Part model, mm, in its own coordinate system. Face numbers are marked on the shaded views. A direction names the side the tool comes from. Give positions to 0.01 mm unless a question says otherwise; leave off trailing zeros. Write each loop counter-clockwise with the first axis right and the second up, starting at its lowest first coordinate (ties: lowest second). Pieces come first, ordered by that corner, then holes. Notation, with made-up numbers: M 0.5,74 L 13.5,74 A25 cw 13.5,107 Z; hole C 38.5,-37.5 d1. An arc over 180 degrees is marked long. Use CSV: the item, a comma, the result in double quotes. Start each with the question number.
1. Band-saw the part on C-C, the plane x = -29.5. List the corners of the cut face in (y, z) (3 decimals), then the cut area to 3 significant figures.
2. Drop flat-ended pins along their axis: pin 1 Ø3 at (y, z) = (14, 5) entering from +X; pin 2 Ø8 at (y, z) = (6, 9.5) entering from +X; pin 3 Ø1 at (y, z) = (-12.5, 13) entering from +X. Give the stop position or say it passes through.
3. 3-axis set-ups, long thin cutter, end or side, ignore diameter. For the marked faces 5 and 6: which of +Z, -Z, +X, -X, +Y, -Y reach the whole face in a straight line?
4. Drill centre lines: line 1 along Z through (x, y) = (0, -15) (3 decimals); line 2 along Y through (x, z) = (9.5, 1.25); line 3 along Z through (x, y) = (-22.5, 0) (3 decimals). Where is each one in solid material? Low to high. Write a range as from..to.
5. Band-saw the part on A-A, the plane z = 3. List the corners of the cut face in (x, y).
6. Mould opens along Z. For the marked faces 1, 2, 3 and 4 say: pulls with the +Z half, pulls with the -Z half, needs draft (parallel to the pull), parting line crosses it, or undercut.
7. Band-saw the part on B-B, the plane x = 0. List the corners of the cut face in (y, z) (3 decimals).
8. Band-saw the part on D-D, the plane z = 10.75. List the corners of the cut face in (x, y), then the cut area to 3 significant figures.
from build123d import *

# Parameters (mm, degrees)
SKETCH_R          = 12.7
SKETCH_R_2        = 2.5
SKETCH_R_3        = 2
PAD_DEPTH         = 9.525
SKETCH001_R       = 18.5
SKETCH001_R_2     = 12.7
PAD001_DEPTH      = 19
SKETCH002_R       = 3.175
POCKET_DEPTH      = 18.501
POCKET_DEPTH_BACK = -18.501
POCKET001_DEPTH   = 3
CHAMFER_SIZE      = 1


with BuildPart() as part:
    # Sketch (on XY_Plane of Origin) → Pad (new body)
    with BuildSketch(Plane.XY):
        with BuildLine():
            ThreePointArc((-46.137289, 5.757869), (-50.45, 0), (-46.137289, -5.757869))
            Line((-46.137289, -5.757869), (-5.202475, -17.753429))
            ThreePointArc((-5.202475, -17.753429), (18.5, 0), (-5.202475, 17.753429))
            Line((-46.137289, 5.757869), (-5.202475, 17.753429))
        make_face()
        Circle(SKETCH_R, mode=Mode.SUBTRACT)
        with Locations((-44.45, 0)):
            Circle(SKETCH_R_2, mode=Mode.SUBTRACT)
        with Locations((-28.57, 0)):
            Circle(SKETCH_R_3, mode=Mode.SUBTRACT)
    extrude(amount=PAD_DEPTH)

    # Sketch001 (on XY_Plane of Origin) → Pad001 (join)
    with BuildSketch(Plane.XY):
        Circle(SKETCH001_R)
        Circle(SKETCH001_R_2, mode=Mode.SUBTRACT)
    extrude(amount=PAD001_DEPTH)

    # Sketch002 (on XZ_Plane of Origin) → Pocket (cut, two sides)
    with BuildSketch(Plane.XZ) as pocket_sk:
        with Locations((0, 9.5)):
            Circle(SKETCH002_R)
    extrude(amount=-POCKET_DEPTH, mode=Mode.SUBTRACT)
    extrude(pocket_sk.sketch, amount=-POCKET_DEPTH_BACK, mode=Mode.SUBTRACT)

    # Sketch003 (on XY_Plane of Origin) → Pocket001 (cut)
    with BuildSketch(Plane.XY.offset(9.53)):
        Polygon((-44.45, 4.618802), (-48.45, 2.309401), (-48.45, -2.309401), (-44.45, -4.618802), (-40.45, -2.309401), (-40.45, 2.309401), align=None)
    extrude(amount=-POCKET001_DEPTH, mode=Mode.SUBTRACT)

    # Chamfer
    chamfer_edges = [part.edges().sort_by_distance(p)[0] for p in [
        (-25.669882, -11.755649, 0),
    ]]
    chamfer(chamfer_edges, length=CHAMFER_SIZE)


solid = part.part
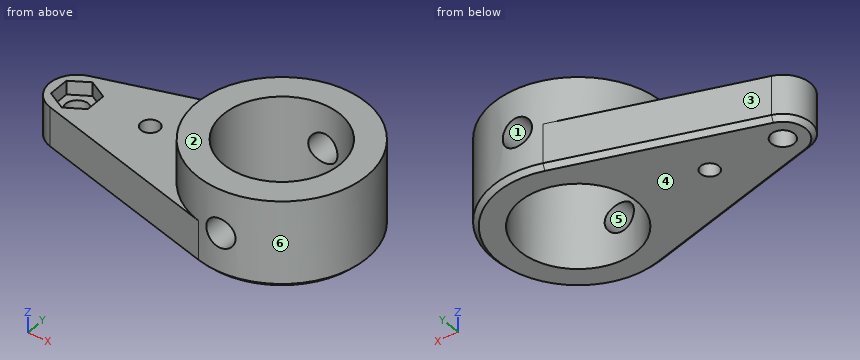
Output:
1,outline,"M -10.633,1 L -9.591,0 L -1.771,0 L -1.771,9.525 L -10.633,9.525 Z; M 1.771,0 L 9.591,0 L 10.633,1 L 10.633,9.525 L 1.771,9.525 Z"
1,area,"168 mm²"
2,pin 1,"stops at x = 13.64"
2,pin 2,"stops at x = 18.39"
2,pin 3,"stops at x = 14.08"
3,face 5,"+Y, -Y"
3,face 6,"+Z"
4,line 1,"z = 0..6.325, 12.675..19"
4,line 2,"y = -15.87..-8.43, 8.43..15.87"
4,line 3,"z = 0..9.525"
5,outline,"M -46.14,-5.76 L -5.21,-17.75 A18.5 ccw long -5.21,17.75 L -46.14,5.76 A6 ccw Z; hole C -44.45,0 d5; hole C -28.57,0 d4; hole C 0,0 d25.4"
6,face 1,"undercut"
6,face 2,"pulls with the +Z half"
6,face 3,"needs draft"
6,face 4,"pulls with the -Z half"
7,outline,"M -18.5,1 L -17.5,0 L -12.7,0 L -12.7,6.325 L -18.5,6.325 Z; M -18.5,12.675 L -12.7,12.675 L -12.7,19 L -18.5,19 Z; M 12.7,0 L 17.5,0 L 18.5,1 L 18.5,6.325 L 12.7,6.325 Z; M 12.7,12.675 L 18.5,12.675 L 18.5,19 L 12.7,19 Z"
8,outline,"M -2.92,-18.27 L -2.92,-12.36 A12.7 cw -2.92,12.36 L -2.92,18.27 A18.5 ccw Z; M 2.92,-18.27 A18.5 ccw 2.92,18.27 L 2.92,12.36 A12.7 cw 2.92,-12.36 Z"
8,area,"500 mm²"
